from build123d import *

# Parameters (mm, degrees)
F0_W         = 80
F0_H         = 50
F1_DEPTH     = 30
F2_T         = -2
F3_R         = 2.2
F3_R_2       = 1
F4_DEPTH     = 5.2
F5_W         = 46
F5_H         = 28
F6_DEPTH     = 25
F7_W         = 2.4
F7_H         = 1.2
F8_DEPTH     = 78
F10_DEPTH    = 8
F11_T1_DEPTH = 13.4474487139
F11_T3_DEPTH = 17.690486541
F12_D        = 2
F12_DEPTH    = 6
F12_TIP      = 0.600860619
F14_DEPTH    = 25


# Not quite as in the source:
# - a fillet or chamfer that OpenCascade refuses, or shapes differently, is made with other operations: its cross-section is extruded or revolved along the edge and cut away or added


with BuildPart() as f1:
    # F0 (on Top) → F1 (new body)
    with BuildSketch(Plane.XY):
        Rectangle(F0_W, F0_H)
    extrude(amount=F1_DEPTH)

    # F2
    f2_openings = [f1.faces().sort_by_distance(p)[0] for p in [
        (0, 0, 30),
    ]]
    offset(amount=F2_T, openings=f2_openings)

    # F3 (on face) → F4 (join)
    with BuildSketch(Plane.XY):
        with Locations((-10.7, 16.75)):
            Circle(F3_R)
        with Locations((-10.7, 16.75)):
            Circle(F3_R_2, mode=Mode.SUBTRACT)
        with Locations((-10.7, -16.75)):
            Circle(F3_R)
        with Locations((-10.7, -16.75)):
            Circle(F3_R_2, mode=Mode.SUBTRACT)
        with Locations((33.8, 16.75)):
            Circle(F3_R)
        with Locations((33.8, 16.75)):
            Circle(F3_R_2, mode=Mode.SUBTRACT)
        with Locations((33.8, -16.75)):
            Circle(F3_R)
        with Locations((33.8, -16.75)):
            Circle(F3_R_2, mode=Mode.SUBTRACT)
    extrude(amount=F4_DEPTH)

    # F5 (on face) → F6 (cut)
    with BuildSketch(Plane.YZ.offset(-38)):
        with Locations((0, 16)):
            Rectangle(F5_W, F5_H)
    extrude(amount=-F6_DEPTH, mode=Mode.SUBTRACT)

    # F7 (on face) → F8 (join, through all)
    with BuildSketch(Plane(origin=(-40, 0, 0), x_dir=(0, -1, 0), z_dir=(-1, 0, 0))):
        Polygon((-20.6, 27.8), (-23, 27.8), (-23, 25), (-20.6, 27.4), align=None)
        Polygon((20.6, 26.8), (23, 24.4), (23, 27.8), (20.6, 27.8), align=None)
        with Locations((21.8, 29.4)):
            Rectangle(F7_W, F7_H)
        with Locations((-21.8, 29.4)):
            Rectangle(F7_W, F7_H)
    extrude(amount=-F8_DEPTH)

    # F9 (on face) → F10 (join)
    with BuildSketch(Plane(origin=(-40, 0, 0), x_dir=(0, -1, 0), z_dir=(-1, 0, 0))):
        Polygon((-21.7, 3.3), (-23, 2), (-19, 2), (-19, 3.2), (-20.4, 4.6), align=None)
        Polygon((-23, 6), (-23, 2), (-21.7, 3.3), (-20.4, 4.6), (-21.8, 6), align=None)
        Polygon((19, 2), (23, 2), (23, 6), (21.8, 6), (19, 3.2), align=None)
    extrude(amount=-F10_DEPTH)

    # F11: fillet of radius 5 on 4 edges, made by hand

    # F11_s2 → F11_t1 (cut)
    with BuildSketch(Plane.XY.offset(2)):
        with BuildLine():
            ThreePointArc((-36.8989794856, 19), (-33.7367018254, 20.1270166538), (-32, 23))
            Line((-32, 23), (-32, 19))
            Line((-32, 19), (-36.8989794856, 19))
        make_face()
        with BuildLine():
            ThreePointArc((-36.8989794856, -19), (-33.7367018254, -20.1270166538), (-32, -23))
            Line((-32, -23), (-32, -19))
            Line((-32, -19), (-36.8989794856, -19))
        make_face()
    extrude(amount=F11_T1_DEPTH, mode=Mode.SUBTRACT)

    # F11_s4 → F11_t3 (cut)
    with BuildSketch(Plane.YZ.offset(-44.8452432705)):
        with BuildLine():
            ThreePointArc((-23, 6), (-21.6127664169, 5.5061172285), (-20.4295582508, 4.6295582508))
            Line((-20.4295582508, 4.6295582508), (-21.8, 6))
            Line((-21.8, 6), (-23, 6))
        make_face()
        with BuildLine():
            ThreePointArc((20.4295582508, 4.6295582508), (21.6127664169, 5.5061172285), (23, 6))
            Line((23, 6), (21.8, 6))
            Line((21.8, 6), (20.4295582508, 4.6295582508))
        make_face()
    extrude(amount=F11_T3_DEPTH, mode=Mode.SUBTRACT)

    # F12
    with Locations(Plane(origin=(-40, 0, 0), x_dir=(0, -1, 0), z_dir=(-1, 0, 0))):
        with Locations((-21.7, 3.3), (21.7, 3.3)):
            Hole(F12_D / 2, depth=F12_DEPTH)
            with Locations((0, 0, -(F12_DEPTH + F12_TIP / 2))):  # 118° drill point
                Cone(0, F12_D / 2, F12_TIP, mode=Mode.SUBTRACT)

    # F13 (on face) → F14 (cut)
    with BuildSketch(Plane.XZ.offset(-23)):
        with BuildLine():
            ThreePointArc((-28, 6), (-17.527864045, 5.05572809), (-12, 14))
            ThreePointArc((-12, 14), (-22, 24), (-32, 14))
            ThreePointArc((-32, 14), (-30.94427191, 9.527864045), (-28, 6))
        make_face()
        with BuildLine():
            ThreePointArc((30, 21.8), (25.2, 17), (30, 12.2))
            Line((30, 12.2), (30, 17))
            Line((30, 17), (30, 21.8))
        make_face()
        with BuildLine():
            ThreePointArc((34.8, 17), (33.3941125497, 20.3941125497), (30, 21.8))
            Line((30, 21.8), (30, 17))
            Line((30, 17), (34.8, 17))
        make_face()
        with BuildLine():
            Line((30, 17), (30, 12.2))
            ThreePointArc((30, 12.2), (33.3941125497, 13.6058874503), (34.8, 17))
            Line((34.8, 17), (30, 17))
        make_face()
    extrude(amount=-F14_DEPTH, mode=Mode.SUBTRACT)


solid = f1.part
Build history of the part. All positions in model axes, mm. A direction names the side the tool comes from. Give positions to 0.01 mm unless a question says otherwise; leave off trailing zeros. Order: outer loops, then holes, each group sorted by start corner. A loop starts at its lowest first (then second) coordinate and runs counter-clockwise, first axis right, second up. Notation, with made-up numbers: M -32,-11.75 L 9,-11.75 A16 cw 9,-1.75 Z; hole C 21,32 d8. An arc over 180 degrees is marked long. Use one line per item in the form item = value.
1) Saw through at B-B (x = -22.5). Give the cut face in (y, z).
Calculated:
outline = M -25,0 L 25,0 L 25,4.01 L 23,4.01 L 23,2 L -23,2 L -23,24.4 L -20.6,26.8 L -20.6,27.8 L -23,27.8 L -23,28.8 L -20.6,28.8 L -20.6,30 L -25,30 Z; M 20.6,27.4 L 23,25 L 23,23.99 L 25,23.99 L 25,30 L 20.6,30 L 20.6,28.8 L 23,28.8 L 23,27.8 L 20.6,27.8 Z
2) Two-plate mould, pull along Z, no slides. Class faces 4 (the face through (-1, 0, 0)), 5 (the face through (-1, 25, 15)), 6 (the face through (-36.1, -21.6, 5.5)): released by +Z, released by -Z, zero draft, split by the parting line, or undercut.
Calculated:
face_4 = released by -Z
face_5 = zero draft
face_6 = undercut
3) Saw through at D-D (x = 12.5). Give the cut face in (y, z), plus the area to 3 significant figures.
Calculated:
outline = M -25,0 L 25,0 L 25,30 L 20.6,30 L 20.6,28.8 L 23,28.8 L 23,27.8 L 20.6,27.8 L 20.6,27.4 L 23,25 L 23,2 L -23,2 L -23,24.4 L -20.6,26.8 L -20.6,27.8 L -23,27.8 L -23,28.8 L -20.6,28.8 L -20.6,30 L -25,30 Z
area = 227 mm2
4) Probe probe 1 along X at (y, z) = (-16.75, 4.25); probe 2 along Y at (x, z) = (33.8, 4.15); probe 3 along Y at (x, z) = (-33.5, 7.75). List the from-to ranges inside material, lowest first.
Calculated:
probe_1 = -12.9 to -11.7, -9.7 to -8.5, 31.6 to 32.8, 34.8 to 36, 38 to 40
probe_2 = -25 to -23, -18.95 to -17.75, -15.75 to -14.55, 14.55 to 15.75, 17.75 to 18.95, 23 to 25
probe_3 = -25 to -23, 23 to 25
5) Saw through at A-A (z = 14). Give the cut face in (x, y), plus the area to 3 significant figures.
Calculated:
outline = M -40,-25 L 40,-25 L 40,25 L 33.75,25 L 33.75,23 L 38,23 L 38,-23 L -40,-23 Z; M -40,23 L -32,23 L -32,25 L -40,25 Z; M -12,23 L 26.25,23 L 26.25,25 L -12,25 Z
area = 357 mm2
6) Saw through at C-C (y = 16.75). Give the cut face in (x, z).
Calculated:
outline = M -40,0 L 40,0 L 40,30 L 38,30 L 38,2 L 36,2 L 36,5.2 L 34.8,5.2 L 34.8,2 L 32.8,2 L 32.8,5.2 L 31.6,5.2 L 31.6,2 L -8.5,2 L -8.5,5.2 L -9.7,5.2 L -9.7,2 L -11.7,2 L -11.7,5.2 L -12.9,5.2 L -12.9,2 L -40,2 Z
7) Drop flat-ended pins along their axis: pin 1 (3 mm diameter, centred on x = -24, z = 16.5, fed in from +Y); pin 2 (14 mm diameter, centred on y = 8.5, z = 16.5, fed in from -X); pin 3 (23 mm diameter, centred on x = 4, y = -1.5, fed in from +Z). Give the stop position or say it passes through.
Calculated:
pin_1 = -23
pin_2 = 38
pin_3 = 2
8) Tool access for faces 1 (the face through (0, -23, 13)), 2 (the face through (35, 16, 5.2)), 3 (the face through (-2, -22, 27.8)): list every direction of +Z, -Z, +X, -X, +Y, -Y with a clear straight run to the whole face (end or side of a thin tool).
Calculated:
face_1 = none
face_2 = +Z, -X
face_3 = -X
